Autodesk Inventor part; units mm, degrees
ref_plane "YZ Plane" through (0, 0, 0) normal (1, 0, 0) x (0, 1, 0)
ref_plane "XZ Plane" through (0, 0, 0) normal (0, 1, 0) x (-1, 0, 0)
ref_plane "XY Plane" through (0, 0, 0) normal (0, 0, 1) x (1, 0, 0)
sketch "스케치1" plane through (0, 0, 0) normal (0, 1, 0) x (-1, 0, 0)
  line L0 (28.5, 0) -> (-28.5, 0)
  line L1 (-26.25, 0) -> (-30.75, 0)
  circle A0 centre (-28.5, 0) radius 10
  line L2 (0, -98.6) -> (0, 28.1)
  line L3 (53.9, 0) -> (-53.9, 0)
  circle A1 centre (28.5, 0) radius 10
  line L4 (20.25, -70.5) -> (-20.25, -70.5)
  circle A2 centre (-20.25, -70.5) radius 10
  circle A3 centre (-20.25, -70.5) radius 3.25
  circle A4 centre (20.25, -70.5) radius 10
  line L5 (30.1822, -71.6623) -> (38.4322, -1.1623)
  line L6 (20.25, -80.5) -> (-20.25, -80.5)
  line L7 (28.5, 10) -> (-28.5, 10)
  line L8 (-30.1822, -71.6623) -> (-38.4322, -1.1623)
  line L9 (10.3178, -69.3377) -> (18.5678, 1.1623)
  line L10 (20.25, -60.5) -> (-20.25, -60.5)
  line L11 (-10.3178, -69.3377) -> (-18.5612, 1.1063)
  line L12 (27.5, -10) -> (-28.5, -10)
  circle A5 centre (-28.5, 0) radius 3.25
  circle A6 centre (20.25, -70.5) radius 3.25
  circle A7 centre (28.5, 0) radius 3.25
  point P0 (0, 0)
  point P1 (0, 0)
  point P2 (0, -70.5)
  point P3 (-17, -70.5)
  point P4 (-23.5, -70.5)
  point P5 (18.5, 0)
  point P6 (18.4318, 0)
  point P7 (-18.0599, 1.0927)
  point P8 (-18.4318, 0)
  point P9 (-18.5, 0)
  point P10 (-11.352, -60.5)
  point P11 (-17.2616, -10)
  point P12 (17.2616, -10)
  point P13 (11.352, -60.5)
  dimension "d0" = 57
  dimension "d7" = 20
  dimension "d10" = 40.5
  dimension "d11" = 70.5
  dimension "d12" = 20
  dimension "d13" = 6.5
  dimension "d17" = 6.5
  dimension "d18" = 6.5
  dimension "d19" = 6.5
extrude "돌출1" add sketch "스케치1" along normal blind 7 contours A0 L3 A5 L0 | A0 L11 L0 | L0 A5 L3 A0 | L0 L11 L12 A0 | L11 A0 L7 L2 L0 | L0 L2 L12 L11 | L12 L11 L10 A2 L8 A0 | L2 L7 A1 L9 L0 | L0 L9 L12 L2 | L9 A1 L0 | L0 A1 L5 A4 L10 L9 | L11 A2 L10 | L10 L2 L4 A2 L11 | A2 | A1 L3 A7 L0 | L0 A7 L3 A1 | L10 L9 A4 L4 L2 | A2 L4 L2 L6 | L10 A4 L9 | L4 A4 L6 L2 | A4
sketch "스케치2" plane through (0, 7, 0) normal (0, 1, 0) x (1, 0, 0)
  point P0 (0, 0)
sketch "스케치3" plane through (0, 7, 0) normal (0, 1, 0) x (1, 0, 0)
  circle A0 centre (0, 0) radius 4
  line L0 (-30.1822, 71.6623) -> (-38.4322, 1.1623)
  arc A1 (-38.4322, 1.1623) -> (-28.5, -10) centre (-28.5, 0) ccw
  line L1 (-28.5, -10) -> (28.5, -10)
  arc A2 (28.5, -10) -> (38.4322, 1.1623) centre (28.5, 0) ccw
  line L2 (38.4322, 1.1623) -> (30.1822, 71.6623)
  arc A3 (30.1822, 71.6623) -> (20.25, 80.5) centre (20.25, 70.5) ccw
  line L3 (20.25, 80.5) -> (-20.25, 80.5)
  arc A4 (-20.25, 80.5) -> (-30.1822, 71.6623) centre (-20.25, 70.5) ccw
  circle A5 centre (20.25, 70.5) radius 3.25
  line L4 (11.352, 60.5) -> (17.2616, 10)
  line L5 (17.2616, 10) -> (-17.2616, 10)
  line L6 (-17.2616, 10) -> (-11.352, 60.5)
  line L7 (-11.352, 60.5) -> (11.352, 60.5)
  circle A6 centre (28.5, 0) radius 3.25
  circle A7 centre (-28.5, 0) radius 3.25
  circle A8 centre (-20.25, 70.5) radius 3.25
  line L8 (0, 0) -> (0, 45)
  line L9 (-23, 45) -> (23, 45)
  circle A9 centre (-23, 45) radius 4
  circle A10 centre (23, 45) radius 4
  line L10 (-2, 3.4641) -> (2, 3.4641)
  line L11 (-2, 3.4641) -> (-4, 0)
  line L12 (57.3115, 0) -> (-57.3115, 0)
  line L13 (-4, 0) -> (-2, -3.4641)
  line L14 (-2, -3.4641) -> (2, -3.4641)
  line L15 (4, 0) -> (2, -3.4641)
  line L16 (4, 0) -> (2, 3.4641)
  line L17 (-25, 48.4641) -> (-21, 48.4641)
  line L18 (-25, 48.4641) -> (-27, 45)
  line L19 (-21, 48.4641) -> (-19, 45)
  line L20 (-19, 45) -> (-21, 41.5359)
  line L21 (-25, 41.5359) -> (-21, 41.5359)
  line L22 (-25, 41.5359) -> (-27, 45)
  line L23 (25, 48.4641) -> (21, 48.4641)
  line L24 (25, 48.4641) -> (27, 45)
  line L25 (21, 48.4641) -> (19, 45)
  line L26 (19, 45) -> (21, 41.5359)
  line L27 (25, 41.5359) -> (21, 41.5359)
  line L28 (25, 41.5359) -> (27, 45)
  circle A11 centre (-23, 45) radius 2
  circle A12 centre (23, 45) radius 2
  circle A13 centre (0, 0) radius 2
  dimension "d20" = 8
  dimension "d21" = 45
  dimension "d22" = 46
  dimension "d23" = 8
  dimension "d24" = 8
  dimension "d25" = 4
  dimension "d26" = 4
  dimension "d27" = 4
  dimension "d28" = 4
  dimension "d31" = 4
  dimension "d32" = 4
  dimension "d33" = 4
extrude "돌출2" cut sketch "스케치3" against normal blind 3 contours L15 L14 L13 L12 A13 | A11 | L20 L21 L22 L18 L17 L19 | A12 | L25 L23 L24 L28 L27 L26 | L12 A13 L8 L10 L16 | A13 L12 | L12 L8 A13 | L8 A13 L12 L11 L10 | L12 A13 L8
extrude "돌출3" cut sketch "스케치3" against normal blind 7 contours A11 | A12 | A13 L12 | L12 L8 A13 | L12 A13 L8
properties part number "라이다"
Model file for the job. Use its own axes, mm. A direction names the side the tool comes from. Coordinates: 2 decimals unless noted, no trailing zeros. Write each loop counter-clockwise with the first axis right and the second up, starting at its lowest first coordinate (ties: lowest second). Pieces come first, ordered by that corner, then holes. Notation, with made-up numbers: (53, -29) -> (93, -29) arc R12 ccw to (93, -13) -> close; hole circle Ø7 at (-13.75, 51). An arc over 180 degrees is marked (long way). One line per item, written item: value. Start each with the question number.
1) Slice it at A-A on x = 8.5. Write the cut outline in (y, z), then the cut area to 3 significant figures.
2) Slice it at D-D on z = -70.5. Write the cut outline in (x, y), then the cut area to 3 significant figures.
3) Pull direction X, two halves, no side cores. Call faces 1 (the face through (0, 3, 10)), 2 (the face through (36.05, 3.45, 6.56)), 3 (the face through (-21, 4, -47)): +X half, -X half, draft (parallel to the pull), parting line (faces both ways), or undercut.
4) Which spindle directions (+Z, -Z, +X, -X, +Y, -Y) get a long thin tool onto all of the face, cutting with end or side? Do faces 4 (the face through (0, 3, -60.5)), 5 (the face through (-25.986, 5.521, -46.756)), 6 (the face through (-17, 0, -35)). Say none if no direction does.
5) Flat gauge pins, fed straight in: pin 1 Ø1 at (y, z) = (2.5, -44) entering from -X; pin 2 Ø3.5 at (x, y) = (-23.5, 6) entering from -Z. Where does each tip first touch, or does it go through?
6) Probe probe 1 along X at (y, z) = (3.75, 0); probe 2 along Z at (x, y) = (-2, 6.75); probe 3 along Z at (x, y) = (-20.25, 2). List the from-to ranges inside material, lowest first.
7) Slice it at B-B on y = 6. Count the separate pieces of the cut face and the enclosed holes in it, then the cut area to 3 significant figures.
8) Slice it at C-C on z = -16.5. Write the cut outline in (x, y).
Answers follow:
1. outline: (0, -80.5) -> (7, -80.5) -> (7, -60.5) -> (0, -60.5) -> close; (0, -10) -> (7, -10) -> (7, 10) -> (0, 10) -> close
1. area: 280 mm2
2. outline: (-30.32, 0) -> (-23.5, 0) -> (-23.5, 7) -> (-30.32, 7) -> close; (-17, 0) -> (17, 0) -> (17, 7) -> (-17, 7) -> close; (23.5, 0) -> (30.32, 0) -> (30.32, 7) -> (23.5, 7) -> close
2. area: 333 mm2
3. face 1: draft
3. face 2: +X half
3. face 3: undercut
4. face 4: +Y, -Y
4. face 5: +Y
4. face 6: +Z, -Z, +X, -X, -Y
5. pin 1: x = -33.48
5. pin 2: z = -80.39
6. probe 1: -38.5 to -31.75, -25.25 to -2, 2 to 25.25, 31.75 to 38.5
6. probe 2: -80.5 to -60.5, -10 to -3.46, 3.46 to 10
6. probe 3: -80.5 to -73.75, -67.25 to 10
7. separate pieces: 1
7. enclosed holes: 8
7. area: 4,440 mm2
8. outline: (-36.64, 0) -> (-16.5, 0) -> (-16.5, 7) -> (-36.64, 7) -> close; (16.5, 0) -> (36.64, 0) -> (36.64, 7) -> (16.5, 7) -> close
